from build123d import *

# Parameters (mm, degrees)
SKETCH_1_W          = 40
SKETCH_1_H          = 15
EXTRUDE_1_DEPTH     = 50
SKETCH_2_W          = 20
SKETCH_2_H          = 50
CUT_EXTRUDE_1_DEPTH = 16
FILLET_2_R          = 5
FILLET_3_R          = 5
CUT_EXTRUDE_2_DEPTH = 4.5
SKETCH_5_W          = 23.5
SKETCH_5_H          = 12.4
CUT_EXTRUDE_3_DEPTH = 18.5
SKETCH_7_W          = 12.4
SKETCH_7_H          = 8
CUT_EXTRUDE_4_DEPTH = 9.25
CUT_EXTRUDE_7_DEPTH = 12


with BuildPart() as part:
    # 스케치1 → 보스-돌출1 (new body, symmetric)
    with BuildSketch(Plane(origin=(0, 0, 0), x_dir=(1, 0, 0), z_dir=(0, 1, 0))):
        Rectangle(SKETCH_1_W, SKETCH_1_H)
    extrude(amount=EXTRUDE_1_DEPTH, both=True)

    # 스케치2 → 컷-돌출1 (cut, through all)
    with BuildSketch(Plane.XY.offset(7.5)):
        with Locations((-10, -25)):
            Rectangle(SKETCH_2_W, SKETCH_2_H)
    extrude(amount=-CUT_EXTRUDE_1_DEPTH, mode=Mode.SUBTRACT)

    # 필렛2
    fillet_2_edges = [part.edges().sort_by_distance(p)[0] for p in [
        (-20, 0, 0),
        (0, 0, 0),
    ]]
    fillet(fillet_2_edges, radius=FILLET_2_R)

    # 필렛3
    fillet_3_edges = [part.edges().sort_by_distance(p)[0] for p in [
        (0, -50, 0),
    ]]
    fillet(fillet_3_edges, radius=FILLET_3_R)

    # 스케치4 → 컷-돌출2 (cut)
    with BuildSketch(Plane(origin=(0, 50, 0), x_dir=(1, 0, 0), z_dir=(0, 1, 0))):
        Polygon((16.4, 6.2), (-16.3, 6.2), (-16.3, -6.3), (16.3, -6.3), align=None)
    extrude(amount=-CUT_EXTRUDE_2_DEPTH, mode=Mode.SUBTRACT)

    # 스케치5 → 컷-돌출3 (cut)
    with BuildSketch(Plane(origin=(0, 45.5, 0), x_dir=(1, 0, 0), z_dir=(0, 1, 0))):
        Rectangle(SKETCH_5_W, SKETCH_5_H)
    extrude(amount=-CUT_EXTRUDE_3_DEPTH, mode=Mode.SUBTRACT)

    # 스케치7 → 컷-돌출4 (cut, through all)
    with BuildSketch(Plane.ZY.offset(-11.75)):
        with Locations((0, 31)):
            Rectangle(SKETCH_7_W, SKETCH_7_H)
    extrude(amount=-CUT_EXTRUDE_4_DEPTH, mode=Mode.SUBTRACT)

    # 스케치10 → 컷-돌출7 (cut)
    with BuildSketch(Plane(origin=(0, 45.5, 0), x_dir=(1, 0, 0), z_dir=(0, 1, 0))):
        Polygon((13.75, -6.3), (13.75, 6.2), (11.75, 6.2), (11.75, -6.2), (11.75, -6.3), align=None)
    extrude(amount=-CUT_EXTRUDE_7_DEPTH, mode=Mode.SUBTRACT)


solid = part.part
Input: part model. Units: mm. Frame: model coordinates. A direction names the side the tool comes from. Give positions to 0.01 mm unless a question says otherwise; leave off trailing zeros. Order: outer loops, then holes, each group sorted by start corner. A loop starts at its lowest first (then second) coordinate and runs counter-clockwise, first axis right, second up. Notation, with made-up numbers: (-36, -13.75) - (9, -13.75) arc R22 cw to (9, 8.25) - close; hole circle Ø10 at (18.25, 32). An arc over 180 degrees is marked (long way). Write each question's results on one line, items separated by ' | '.
Item 1: Section C-C (x = -6). Return loops of the section in (y, z), and give its area (3 significant figures).
A:
outline: (0, -7.5) - (50, -7.5) - (50, -6.2) - (27, -6.2) - (27, 6.2) - (45.5, 6.2) - (45.5, 6.3) - (50, 6.3) - (50, 7.5) - (0, 7.5) - close | area: 464 mm^2
Item 2: Section D-D (z = 3.75). Return loops of the section in (x, y).
A:
outline: (-20, 5) arc R5 ccw to (-15, 0) - (-5, 0) arc R5 cw to (0, -5) - (0, -45) arc R5 ccw to (5, -50) - (20, -50) - (20, 27) - (-11.75, 27) - (-11.75, 45.5) - (-16.3, 45.5) - (-16.3, 50) - (-20, 50) - close; (13.75, 35) - (20, 35) - (20, 50) - (16.32, 50) - (16.32, 45.5) - (13.75, 45.5) - close
Item 3: Access query for faces 1 (the flat face through (12, -50, 0)), 2 (the flat face through (-10, 0, 0)), 3 (the flat face through (15, 45.5, 0)), 4 (the flat face through (17, 35, 0)). Directions: +Z, -Z, +X, -X, +Y, -Y. A direction counts if a zero-diameter tool reaches every point of the face in a straight line with its end or side. Return the directions, or none.
A:
face 1: +Z, -Z, +X, -X, -Y | face 2: +Z, -Z, -X, -Y | face 3: +Y | face 4: +X
Item 4: Contact query for flat-ended pins moving along their axis: pin 1 Ø6 at (y, z) = (-11, 1) entering from -X; pin 2 Ø1.3 at (x, z) = (15, 3) entering from +Y; pin 3 Ø1 at (y, z) = (-1, -2) entering from -X. Output: stop coordinate, or through.
A:
pin 1: stops at x = 0 | pin 2: stops at y = 45.5 | pin 3: stops at x = -2.82
Item 5: Section A-A (z = -2.5). Return loops of the section in (x, y).
A:
outline: (-20, 5) arc R5 ccw to (-15, 0) - (-5, 0) arc R5 cw to (0, -5) - (0, -45) arc R5 ccw to (5, -50) - (20, -50) - (20, 27) - (-11.75, 27) - (-11.75, 45.5) - (-16.3, 45.5) - (-16.3, 50) - (-20, 50) - close; (13.75, 35) - (20, 35) - (20, 50) - (16.37, 50) - (16.37, 45.5) - (13.75, 45.5) - close
Item 6: Draft query along X for faces 5 (the flat face through (-16.3, 48, 0)), 6 (the flat face through (4, 12, 7.5)), 7 (the flat face through (-20, 28, 0)), 8 (the flat face through (20, 1, 0)). Return one class per face: released by +X, released by -X, zero draft, split by the parting line, or undercut.
A:
face 5: undercut | face 6: zero draft | face 7: released by -X | face 8: released by +X
Item 7: Section B-B (y = 40). Return loops of the section in (x, z), and give its area (3 significant figures).
A:
outline: (-20, -7.5) - (20, -7.5) - (20, 7.5) - (-20, 7.5) - close; hole (-11.75, -6.2) - (13.75, -6.2) - (13.75, 6.3) - (11.75, 6.3) - (11.75, 6.2) - (-11.75, 6.2) - close | area: 284 mm^2
Item 8: Material intervals for line 1 along X through (y, z) = (38.5, 6.25); line 2 along Y through (x, z) = (18, 5.5); line 3 along Z through (x, y) = (3, 30), sorted ascending.
A:
line 1: x = -20 to 11.75, 13.75 to 20 | line 2: y = -50 to 27, 35 to 50 | line 3: z = -7.5 to -6.2, 6.2 to 7.5
